Autodesk Inventor part; units mm, degrees
ref_plane "YZ Plane" through (0, 0, 0) normal (1, 0, 0) x (0, 1, 0)
ref_plane "XZ Plane" through (0, 0, 0) normal (0, 1, 0) x (-1, 0, 0)
ref_plane "XY Plane" through (0, 0, 0) normal (0, 0, 1) x (1, 0, 0)
sketch "スケッチ2" plane through (0, 0, 0) normal (0, 0, 1) x (1, 0, 0)
  line L0 (44, -27.5) -> (-44, -27.5)
  line L1 (-44, -27.5) -> (-44, 27.5)
  line L2 (-44, 27.5) -> (44, 27.5)
  line L3 (44, 27.5) -> (44, -27.5)
  line L4 (44, -27.5) -> (-44, 27.5) construction
  line L5 (-44, -27.5) -> (44, 27.5) construction
  point P0 (0, 0)
  dimension "d5" = 88
  dimension "d6" = 55
extrude "プレート2" add sketch "スケッチ2" along normal blind 2
sketch "スケッチ3" plane through (42, 27.5, 0) normal (1, 0, 0) x (0, 1, 0)
  line L0 (-55, 0) -> (0, 0)
  line L1 (0, 0) -> (0, 30)
  line L2 (0, 30) -> (-55, 30)
  line L3 (-55, 30) -> (-55, 0)
edge flange "フランジ1" height 30 angle 90 thickness 2 bend radius 2 thickness toward (1, 0, 0) relief tear relief width 2 relief depth 1 corner gap 2 corner form 0 edges at (44, 0, 2) (-44, 0, 2) wall of the first edge with corners at (42, -27.5, 0) (42, 27.5, 0) (42, 27.5, 30) (42, -27.5, 30)
bend "曲げ1"
corner "コーナー1"
sketch "スケッチ5" plane through (-44, -27.5, 30) normal (-1, 0, 0) x (0, 0, 1)
  circle A0 centre (17.5, 27.5) radius 37.5
  circle A1 centre (-11.2267, 3.3955) radius 1.8919
  circle A2 centre (10.9882, -9.4303) radius 1.8919
  circle A3 centre (36.25, -4.976) radius 1.8919
  circle A4 centre (52.7385, 14.6742) radius 1.8919
  circle A5 centre (52.7385, 40.3258) radius 1.8919
  circle A6 centre (36.25, 59.976) radius 1.8919
  circle A7 centre (10.9882, 64.4303) radius 1.8919
  circle A8 centre (-11.2267, 51.6045) radius 1.8919
  circle A9 centre (-20, 27.5) radius 1.8919
  line L0 (-26, 55) -> (-26, 0)
  circle A10 centre (17.5, 27.5) radius 30.5
  point P0 (-30, 27.5)
  dimension "d26" = 75
  dimension "d29" = 360
  dimension "d31" = 0
  dimension "d32" = 0
  dimension "d36" = 6
  dimension "d37" = 61
extrude "押し出し1" cut sketch "スケッチ5" against normal up to surface (88 mm away) contours A8 A0 | A0 A8 | A1 A0 | A0 A1 | A9 A0 | A0 A9 | A10
equation "\"d7\" = Thickness"
equation "\"d8\" = BendReliefWidth"
equation "\"d9\" = BendReliefDepth"
equation "\"d10\" = MinimumRemnant"
equation "\"d11\" = TransitionRadius"
equation "\"d14\" = BendRadius"
equation "\"d15\" = CornerReliefSize"
equation "\"d16\" = GapSize"
equation "\"d17\" = JacobiRadiusSize"
equation "\"BendRadius\" = Thickness"
equation "\"BendReliefWidth\" = Thickness"
equation "\"BendReliefDepth\" = 0.5 * Thickness"
equation "\"CornerReliefSize\" = 4 * Thickness"
equation "\"MinimumRemnant\" = 2 * Thickness"
equation "\"TransitionRadius\" = BendRadius"
equation "\"JacobiRadiusSize\" = BendRadius"
equation "\"GapSize\" = Thickness"
properties part number "servo_arm" material "アルミニウム 5052"
For this review, take the finished solid that the model builds, in its own axes (mm). A direction names the side the tool comes from. Give positions to 0.01 mm unless a question says otherwise; leave off trailing zeros. Loops run counter-clockwise (first coordinate to the right, second up) from the corner with the lowest first, then second, coordinate; pieces in that order, holes last. Notation, with made-up numbers: M 11,61.5 L 40,61.5 A28 ccw 40,98.5 Z; hole C -23.5,-30.5 d10. An arc over 180 degrees is marked long. One line per item, written item: value. Start each with the question number.
Q1. Add section D-D (y = -16.5). Give the boundary of the cut face in (x, z).
Q2. Add section B-B (y = 0). Give the boundary of the cut face in (x, z).
Q3. Add section A-A (z = 10). Give the boundary of the cut face in (x, y).
Q4. Draft analysis for pull direction X (two halves, no side actions). For faces 3 (the face through (42.986, 0.568, 11.805)), 4 (the face through (-1, 0, 2)), 5 (the face through (42.859, 0.385, 1.203)), state which applies: released by +X, released by -X, zero draft, split by the parting line, or undercut.
Q5. Clearance check with flat-ended pins moving along their axes: pin 1 Ø5 at (x, y) = (-32, -14) entering from +Z; pin 2 Ø2.5 at (y, z) = (0, 10) entering from -X. State where each tip first meets the part, or that it passes through.
Q6. Add section C-C (z = 18.5). Count the separate pieces of the cut face and the enclosed holes in it, and give its area (3 significant figures).
Q7. For L1, parallel to X at y = -23.5, z = 14; L2, parallel to Y at x = 43, z = 10; L3, parallel to Z at x = -32, y = 20.5, list the stretches that pass through material, from the lowest coordinate up.
Q8. Machinability: for faces 1 (the face through (-43.014, 0.568, 11.805)), 2 (the face through (42, 0, 14)), which of the approach directions +Z, -Z, +X, -X, +Y, -Y give a long, thin tool a straight path to every point of the face, cutting with its end or side? Answer none if there is none.
Reply:
1. outline: M -44,4 A4 ccw -40,0 L 40,0 A4 ccw 44,4 L 44,21.85 L 42,21.85 L 42,4 A2 cw 40,2 L -40,2 A2 cw -42,4 L -42,21.85 L -44,21.85 Z
2. outline: M -44,4 A4 ccw -40,0 L 40,0 A4 ccw 44,4 L 44,8.11 L 42,8.11 L 42,4 A2 cw 40,2 L -40,2 A2 cw -42,4 L -42,8.11 L -44,8.11 Z; M -44,11.89 L -42,11.89 L -42,17 L -44,17 Z; M 42,11.89 L 44,11.89 L 44,17 L 42,17 Z
3. outline: M -44,-27.5 L -42,-27.5 L -42,-1.89 L -44,-1.89 Z; M -44,1.89 L -42,1.89 L -42,27.5 L -44,27.5 Z; M 42,-27.5 L 44,-27.5 L 44,-1.89 L 42,-1.89 Z; M 42,1.89 L 44,1.89 L 44,27.5 L 42,27.5 Z
4. face 3: zero draft
4. face 4: undercut
4. face 5: released by +X
5. pin 1: z = 2
5. pin 2: through
6. separate pieces: 8
6. enclosed holes: 0
6. area: 114 mm²
7. L1: -44 to -42, 42 to 44
7. L2: -27.5 to -1.89, 1.89 to 27.5
7. L3: 0 to 2
8. face 1: +X, -X
8. face 2: +Z, +Y, -Y
